```python
from build123d import *

# Parameters (mm, degrees)
SKETCH046_R         = 26.5
SKETCH046_R_2       = 8.5
SKETCH046_R_3       = 1.65
PAD029_DEPTH        = 8
SKETCH048_R         = 10.5
POCKET014_DEPTH     = 6
HOLE003_D           = 3.4
HOLE003_CBORE_D     = 5.5
HOLE003_CBORE_DEPTH = 4
HOLE004_D           = 3.4
HOLE004_CBORE_D     = 5.5
HOLE004_CBORE_DEPTH = 4
CHAMFER016_SIZE     = 0.75


with BuildPart() as part:
    # Sketch046 → Pad029 (new body)
    with BuildSketch(Plane.YZ.offset(69)):
        with Locations((-10, -6)):
            Circle(SKETCH046_R)
        with Locations((-10, -6)):
            Circle(SKETCH046_R_2, mode=Mode.SUBTRACT)
        with Locations((-10, 9)):
            Circle(SKETCH046_R_3, mode=Mode.SUBTRACT)
        with Locations((2.990381, -13.5)):
            Circle(SKETCH046_R_3, mode=Mode.SUBTRACT)
        with Locations((-22.990381, -13.5)):
            Circle(SKETCH046_R_3, mode=Mode.SUBTRACT)
    extrude(amount=PAD029_DEPTH)

    # Sketch048 → Pocket014 (cut)
    with BuildSketch(Plane.YZ.offset(69)):
        with Locations((-10, -6)):
            Circle(SKETCH048_R)
    extrude(amount=POCKET014_DEPTH, mode=Mode.SUBTRACT)

    # Hole003 (through all)
    with Locations(Plane(origin=(69, 0, 0), x_dir=(0, 1, 0), z_dir=(-1, 0, 0))):
        with Locations((-29.052559, -5), (9.052559, -5), (-10, 28)):
            CounterBoreHole(HOLE003_D / 2, HOLE003_CBORE_D / 2, HOLE003_CBORE_DEPTH)

    # Hole004 (through all)
    with Locations(Plane.YZ.offset(77)):
        with Locations((-22.990381, -13.5), (-10, 9), (2.990381, -13.5)):
            CounterBoreHole(HOLE004_D / 2, HOLE004_CBORE_D / 2, HOLE004_CBORE_DEPTH)

    # Chamfer016
    chamfer016_edges = [part.edges().sort_by_distance(p)[0] for p in [
        (77, -36.5, -6),
    ]]
    chamfer(chamfer016_edges, length=CHAMFER016_SIZE)


with BuildPart() as part_1:
    # Body011 placement: moved
    add(part.part.moved(Location((2, -5.5, 6.5))))


solid = part_1.part
```
The model under review builds one solid part; all positions refer to its coordinate system, in mm. A direction names the side the tool comes from. Give positions to 0.01 mm unless a question says otherwise; leave off trailing zeros. Write each loop counter-clockwise with the first axis right and the second up, starting at its lowest first coordinate (ties: lowest second). Pieces come first, ordered by that corner, then holes. Notation, with made-up numbers: M 41,89 L 47,89 A27 ccw 47,127 Z; hole C 62,54.25 d2. An arc over 180 degrees is marked long. Write item = value, one per line. Start each with the question number.
Q1. Mouldability with a two-part tool opening along Y and no side actions: class faces 1 (the face through (75, -14, -23)), 2 (the face through (79, -22, 7)), 3 (the face through (74.574, 9.776, 8.46)) as released by +Y, released by -Y, zero draft, split by the parting line, or undercut.
Q2. Machinability: for faces 4 (the face through (77.986, -21.765, 6.245)), 5 (the face through (77.028, -31.238, -6.879)), 6 (the face through (75, 2, 13)), which of the approach directions +Z, -Z, +X, -X, +Y, -Y give a long, thin tool a straight path to every point of the face, cutting with its end or side? Answer none if there is none.
Q3. We need section B-B (y = -15.5). Give the number of separate pieces and of enclosed holes in the cut face, plus the area to 3 significant figures.
Q4. Clearance check with flat-ended pins moving along their axes: pin 1 (5 mm diameter, centred on y = -2.51, z = -7, fed in from +X); pin 2 (1.5 mm diameter, centred on x = 78, y = -15, fed in from -Z); pin 3 (4 mm diameter, centred on y = -15.5, z = -21.5, fed in from -X); pin 4 (2 mm diameter, centred on y = -2.51, z = -7, fed in from +X). State where each tip first meets the part, or that it passes through.
Q5. For line 1 (Z direction, x = 73.25, y = -15.5); line 2 (Y direction, x = 72.25, z = 12.5); line 3 (Z direction, x = 72.75, y = -15), list the stretches that pass through material, from the lowest coordinate up.
Q6. We need section A-A (z = 0.5). State the section outline as (x, y) points, plus the area to 3 significant figures.
Result set:
q1.face_1 = undercut
q1.face_2 = zero draft
q1.face_3 = split by the parting line
q2.face_4 = +X, -X
q2.face_5 = +X
q2.face_6 = -X
q3.separate_pieces = 4
q3.enclosed_holes = 0
q3.area = 192 mm2
q4.pin_1 = 75
q4.pin_2 = -26
q4.pin_3 = 75
q4.pin_4 = through
q5.line_1 = -26 to -24.25, -18.75 to -10, 11 to 13.8, 17.2 to 27
q5.line_2 = -39.13 to -37.11, -31.99 to 0.99, 6.11 to 8.13
q5.line_3 = -26 to -24.2, -18.8 to -9.99, 10.99 to 13.88, 17.12 to 27
q6.outline = M 71,-42 L 78.25,-42 L 79,-41.25 L 79,-24 L 77,-24 L 77,-26 L 71,-26 Z; M 71,-5 L 77,-5 L 77,-7 L 79,-7 L 79,10.25 L 78.25,11 L 71,11 Z
q6.area = 263 mm2
